Autodesk Inventor part; units mm, degrees
ref_plane "YZ Plane" through (0, 0, 0) normal (1, 0, 0) x (0, 1, 0)
ref_plane "XZ Plane" through (0, 0, 0) normal (0, 1, 0) x (-1, 0, 0)
ref_plane "XY Plane" through (0, 0, 0) normal (0, 0, 1) x (1, 0, 0)
sketch "Sketch1" plane through (0, 0, 0) normal (0, 0, 1) x (1, 0, 0)
  circle A0 centre (0, 0) radius 10
  circle A1 centre (0, 0) radius 22.5
  line L0 (-22.5, 0) -> (-22.5, -32.5) construction
  line L1 (-22.5, -32.5) -> (22.5, -32.5) construction
  line L2 (22.5, -32.5) -> (22.5, 0) construction
  line L3 (-22.5, 0) -> (-22.5, -22.5)
  line L4 (-22.5, -22.5) -> (-32.5, -22.5)
  line L5 (-32.5, -22.5) -> (-32.5, -32.5)
  line L6 (22.5, 0) -> (22.5, -22.5)
  line L7 (22.5, -22.5) -> (32.5, -22.5)
  line L8 (32.5, -22.5) -> (32.5, -32.5)
  line L9 (32.5, -32.5) -> (-32.5, -32.5)
  dimension "d0" = 20
  dimension "d1" = 45
  dimension "d2" = 22.5
  dimension "d3" = 10
  dimension "d4" = 10
  dimension "d8" = 10
extrude "Extrusion1" add sketch "Sketch1" along normal blind 34
sketch "Sketch2" plane through (32.5, -32.5, 0) normal (1, 0, 0) x (0, 0, -1)
  line L0 (0, 0) -> (-34, 0) construction
  line L1 (0, 55) -> (-34, 55) construction
  line L2 (0, 10) -> (-34, 10) construction
  line L3 (-10, 10) -> (-24, 10)
  line L4 (-24, 10) -> (-24, 55)
  line L5 (-24, 55) -> (-10, 55)
  line L6 (-10, 55) -> (-10, 10)
  line L7 (0, 32.5) -> (-34, 32.5)
  line L8 (-10, 10) -> (-24, 55) construction
  line L9 (-24, 10) -> (-10, 55) construction
  point P0 (-17, 32.5)
  dimension "d9" = 14
extrude "Extrusion2" cut sketch "Sketch2" against normal blind 100
ref_plane "Work Plane1" through (0, 0, 17) normal (0, 0, 1) x (1, 0, 0)
ref_plane "Work Plane2" through (0, -22.5, 34) normal (1, 0, 0) x (0, 0, -1)
properties part number "ApoyoRotatorioPreliminar"
For this review, take the finished solid that the model builds, in its own axes (mm). A direction names the side the tool comes from. Round coordinates to 2 decimals unless told otherwise and drop trailing zeros. Write each loop counter-clockwise with the first axis right and the second up, starting at its lowest first coordinate (ties: lowest second). Pieces come first, ordered by that corner, then holes. Notation, with made-up numbers: (43, -18) -> (89, -18) arc R23 ccw to (89, -9) -> close; hole circle Ø1 at (50, -24). An arc over 180 degrees is marked (long way). Use one line per item in the form item = value.
1) Mouldability with a two-part tool opening along X and no side actions: class faces 4 (the cylindrical face through (-2.17, 9.76, 28.93)), 5 (the flat face through (0, -22.5, 17)), 6 (the flat face through (32.5, -27, 17)) as +X half, -X half, draft (parallel to the pull), parting line (faces both ways), or undercut.
Found:
face_4 = undercut
face_5 = draft
face_6 = +X half
2) Take a section at A-A, the plane z = 30.5. Write out the cut boundary in (x, y), and give its area (3 significant figures).
Found:
outline = (-32.5, -32.5) -> (32.5, -32.5) -> (32.5, -22.5) -> (22.5, -22.5) -> (22.5, 0) arc R22.5 ccw to (-22.5, 0) -> (-22.5, -22.5) -> (-32.5, -22.5) -> close; hole circle Ø20 at (0, 0)
area = 2,140 mm2
3) Take a section at C-C, the plane x = 0. Write out the cut boundary in (y, z).
Found:
outline = (-32.5, 0) -> (-10, 0) -> (-10, 10) -> (-22.5, 10) -> (-22.5, 24) -> (-10, 24) -> (-10, 34) -> (-32.5, 34) -> close; (10, 0) -> (22.5, 0) -> (22.5, 10) -> (10, 10) -> close; (10, 24) -> (22.5, 24) -> (22.5, 34) -> (10, 34) -> close
4) Take a section at D-D, the plane y = -6. Write out the cut boundary in (x, z), and give its area (3 significant figures).
Found:
outline = (-22.5, 0) -> (-8, 0) -> (-8, 10) -> (-22.5, 10) -> close; (-22.5, 24) -> (-8, 24) -> (-8, 34) -> (-22.5, 34) -> close; (8, 0) -> (22.5, 0) -> (22.5, 10) -> (8, 10) -> close; (8, 24) -> (22.5, 24) -> (22.5, 34) -> (8, 34) -> close
area = 580 mm2
5) To check wall thickness, follow L1, parallel to X at y = 0, z = 27; L2, parallel to Z at x = 12.5, y = -9.5; L3, parallel to Y at x = 0, z = 6.75. State the ranges of each line that lie inside material, in increasing order. Write a range as from..to.
Found:
L1 = -22.5..-10, 10..22.5
L2 = 0..10, 24..34
L3 = -32.5..-10, 10..22.5
6) Tool access review of faces 1 (the flat face through (0.3, -10.3, 24)), 2 (the flat face through (-22.5, -11, 29)), 3 (the flat face through (22.5, -11, 5)): name each direction out of +Z, -Z, +X, -X, +Y, -Y from which nothing blocks a thin tool from reaching the whole face with its end or side.
Found:
face_1 = +X, -X, +Y
face_2 = +Z, -Z, -X, +Y
face_3 = +Z, -Z, +X, +Y
7) Take a section at B-B, the plane y = -16.5. Write out the cut boundary in (x, z), and give its area (3 significant figures).
Found:
outline = (-22.5, 0) -> (22.5, 0) -> (22.5, 10) -> (-22.5, 10) -> close; (-22.5, 24) -> (22.5, 24) -> (22.5, 34) -> (-22.5, 34) -> close
area = 900 mm2
8) Clearance check with flat-ended pins moving along their axes: pin 1 (4 mm diameter, centred on x = 16, y = 13.5, fed in from -Z); pin 2 (12 mm diameter, centred on x = 0, y = 0, fed in from -Z); pin 3 (8 mm diameter, centred on y = -16.5, z = 29, fed in from -X); pin 4 (6 mm diameter, centred on y = 8, z = 23, fed in from +X). State where each tip first meets the part, or that it passes through.
Found:
pin_1 = 0
pin_2 = through
pin_3 = -22.5
pin_4 = 21.9
